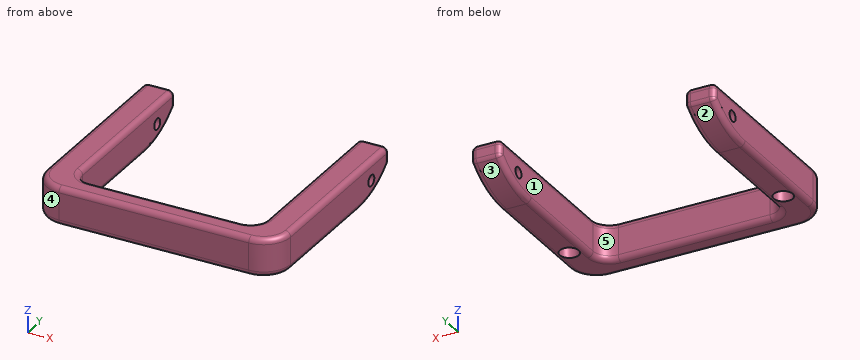
```python
from build123d import *

# Parameters (mm, degrees)
EXTRUDE_1_DEPTH     = 7
SKETCH_3_R          = 1
CUT_EXTRUDE_2_DEPTH = 57.833088954
SKETCH_4_R          = 1.75
CUT_EXTRUDE_3_DEPTH = 2.5
CUT_EXTRUDE_1_DEPTH = 57.833088954
FILLET_2_R          = 15
FILLET_3_R          = 1


# Some blends are built 0.0001 mm under size
with BuildPart() as part:
    # 草图1 → 凸台-拉伸1 (new body)
    with BuildSketch(Plane.XY):
        with BuildLine():
            Line((14, 0), (-14, 0))
            ThreePointArc((-14, 0), (-16.121320344, 0.878679656), (-17, 3))
            Line((-17, 3), (-17, 34))
            Line((-17, 34), (-22.5, 34))
            Line((-22.5, 34), (-22.5, 1))
            ThreePointArc((-22.5, 1), (-21.035533906, -2.535533906), (-17.5, -4))
            Line((-17.5, -4), (17.5, -4))
            ThreePointArc((17.5, -4), (21.035533906, -2.535533906), (22.5, 1))
            Line((22.5, 1), (22.5, 34))
            Line((22.5, 34), (17, 34))
            Line((17, 34), (17, 3))
            ThreePointArc((17, 3), (16.121320344, 0.878679656), (14, 0))
        make_face()
    extrude(amount=EXTRUDE_1_DEPTH)

    # 草图3 → 切除-拉伸2 (cut, through all)
    with BuildSketch(Plane.ZY.offset(22.5)):
        with Locations(Location((3.5, 28, 0), (0, 0, 270))):
            Circle(SKETCH_3_R)
    extrude(amount=-CUT_EXTRUDE_2_DEPTH, mode=Mode.SUBTRACT)

    # 草图4 → 切除-拉伸3 (cut)
    with BuildSketch(Plane(origin=(0, 0, 0), x_dir=(-1, 0, 0), z_dir=(0, 0, -1))):
        with Locations((-19.75, 6)):
            Circle(SKETCH_4_R)
        with Locations(Location((19.75, 6, 0), (0, 0, 180))):
            Circle(SKETCH_4_R)
    extrude(amount=-CUT_EXTRUDE_3_DEPTH, mode=Mode.SUBTRACT)

    # 草图2 → 切除-拉伸1 (cut, through all)
    with BuildSketch(Plane.ZY.offset(22.5)):
        Polygon((0, 30), (4, 34), (7, 34), (7, 35.188575271), (0, 35.188575271), align=None)
    extrude(amount=-CUT_EXTRUDE_1_DEPTH, mode=Mode.SUBTRACT)

    # 圆角2
    # the kernel refuses this fillet: 15 mm, written as the material it takes off along each edge
    with BuildSketch(Plane(origin=(-37.995097568, 30, 0), x_dir=(0, -1, 0), z_dir=(1, 0, 0)), Plane(origin=(1.504902432, 30, 0), x_dir=(0, -1, 0), z_dir=(1, 0, 0))) as fillet_2_piece_1:
        with BuildLine():
            CenterArc((6.198039027, -15), FILLET_2_R, 90, 42.833428066)
            Line((-4, -4), (-4.203960781, -3.78))
            ThreePointArc((-4.203960781, -3.78), (-2.212132034, -1.787867966), (-0.212132034, 0.212132034))
            Line((-0.212132034, 0.212132034), (0, 0.3))
            Line((0, 0.3), (6.198039027, 0.3))
            Line((6.198039027, 0.3), (6.198039027, 0))
        make_face()
    extrude(amount=36.490195136, mode=Mode.SUBTRACT)

    # 圆角3
    fillet_3_edges = [part.edges().sort_by_distance(p)[0] for p in [
        (-17, 13.400980486, 0),
        (-16.121320344, 0.878679656, 0),
        (-21.035533906, -2.535533906, 7),
        (0, 0, 0),
        (16.121320344, 0.878679656, 0),
        (22.5, 12.400980486, 0),
        (21.035533906, -2.535533906, 0),
        (0, -4, 0),
        (-21.035533906, -2.535533906, 0),
        (0, -4, 7),
        (-17, 34, 5.5),
        (21.035533906, -2.535533906, 7),
        (17, 34, 5.5),
        (22.5, 34, 5.5),
        (-22.5, 34, 5.5),
        (22.5, 17.5, 7),
        (19.75, 34, 7),
        (17, 18.5, 7),
        (16.121320344, 0.878679656, 7),
        (0, 0, 7),
        (-16.121320344, 0.878679656, 7),
        (-17, 18.5, 7),
        (-19.75, 34, 7),
        (19.75, 34, 4),
        (-19.75, 34, 4),
        (17, 13.400980486, 0),
        (17, 29.279186548, 1.035759956),
        (-22.5, 12.400980486, 0),
        (22.5, 29.279186548, 1.035759956),
        (-17, 29.279186548, 1.035759956),
        (-22.5, 29.279186548, 1.035759956),
        (-22.5, 17.5, 7),
    ]]
    fillet(fillet_3_edges, radius=FILLET_3_R - 0.0001)  # a hair under: the kernel refuses the full size


solid = part.part
```
Here's how the part is built. I have some questions about the finished solid (model axes, mm). Face numbers are marked on the shaded views. A direction names the side the tool comes from. Round coordinates to 2 decimals unless told otherwise and drop trailing zeros. Order: outer loops, then holes, each group sorted by start corner. A loop starts at its lowest first (then second) coordinate and runs counter-clockwise, first axis right, second up. Notation, with made-up numbers: M 29,83.5 L 44,83.5 A20 ccw 44,90.5 Z; hole C -18,35.5 d5. An arc over 180 degrees is marked long. Answer as CSV lines item,"result".
Item 1: For pin 1 (2.5 mm diameter, centred on y = 28, z = 3.5, fed in from -X); pin 2 (1.5 mm diameter, centred on x = 2.5, z = 4, fed in from +Y); pin 3 (3 mm diameter, centred on x = -19.75, y = 6, fed in from -Z), each with a flat end and sliding along its axis, tell me the tip position at first contact or that it passes through.
From the geometry:
pin 1,"x = -22.5"
pin 2,"y = 0"
pin 3,"z = 2.5"
Item 2: Please list where these lines run through material, in increasing order: L1, parallel to X at y = 26, z = 3; L2, parallel to Y at x = -5.5, z = 2.5; L3, parallel to Z at x = -19, y = 28. Write a range as [from, to].
From the geometry:
L1,"[-22.5, -17], [17, 22.5]"
L2,"[-4, 0]"
L3,"[0.6, 2.5], [4.5, 7]"
Item 3: We'd pull the mould along X, two halves only. Please class the marked faces 3, 4 and 5: +X half, -X half, draft (parallel to the pull), parting line (faces both ways), or undercut.
From the geometry:
face 3,"draft"
face 4,"-X half"
face 5,"undercut"
Item 4: Imagine slicing it at B-B on x = -0.5. List the corners of the cut face in (y, z) for me, and give its area (3 significant figures).
From the geometry:
outline,"M -4,1 A1 ccw -3,0 L -1,0 A1 ccw 0,1 L 0,6 A1 ccw -1,7 L -3,7 A1 ccw -4,6 Z"
area,"27.1 mm2"
Item 5: Imagine slicing it at C-C on z = 3. Give the number of separate pieces and of enclosed holes in the cut face, and give its area (3 significant figures).
From the geometry:
separate pieces,"3"
enclosed holes,"0"
area,"513 mm2"
Item 6: Imagine slicing it at A-A on y = 9. List the corners of the cut face in (x, z) for me, and give its area (3 significant figures).
From the geometry:
outline,"M -22.5,1 A1 ccw -21.5,0 L -18,0 A1 ccw -17,1 L -17,6 A1 ccw -18,7 L -21.5,7 A1 ccw -22.5,6 Z; M 17,1 A1 ccw 18,0 L 21.5,0 A1 ccw 22.5,1 L 22.5,6 A1 ccw 21.5,7 L 18,7 A1 ccw 17,6 Z"
area,"75.3 mm2"
Item 7: Which directions (+Z, -Z, +X, -X, +Y, -Y) give clear straight access to the entire face, cutting with the end or side of a thin tool? Please do the marked faces 1 and 2.
From the geometry:
face 1,"+Z, -Z, +Y"
face 2,"-Z, +X, -X, +Y"
